The figure shows three views and two pictorial views of one solid part (mm, origin at its lowest corner). Answer the questions. A direction names the side the tool comes from. Round coordinates to 2 decimals unless told otherwise and drop trailing zeros. Write each loop counter-clockwise with the first axis right and the second up, starting at its lowest first coordinate (ties: lowest second). Pieces come first, ordered by that corner, then holes. Notation, with made-up numbers: M 83.25,33 L 134.25,33 A25 cw 134.25,46 Z; hole C 49,58 d7. An arc over 180 degrees is marked long. Answer in a Markdown table with one row per item.
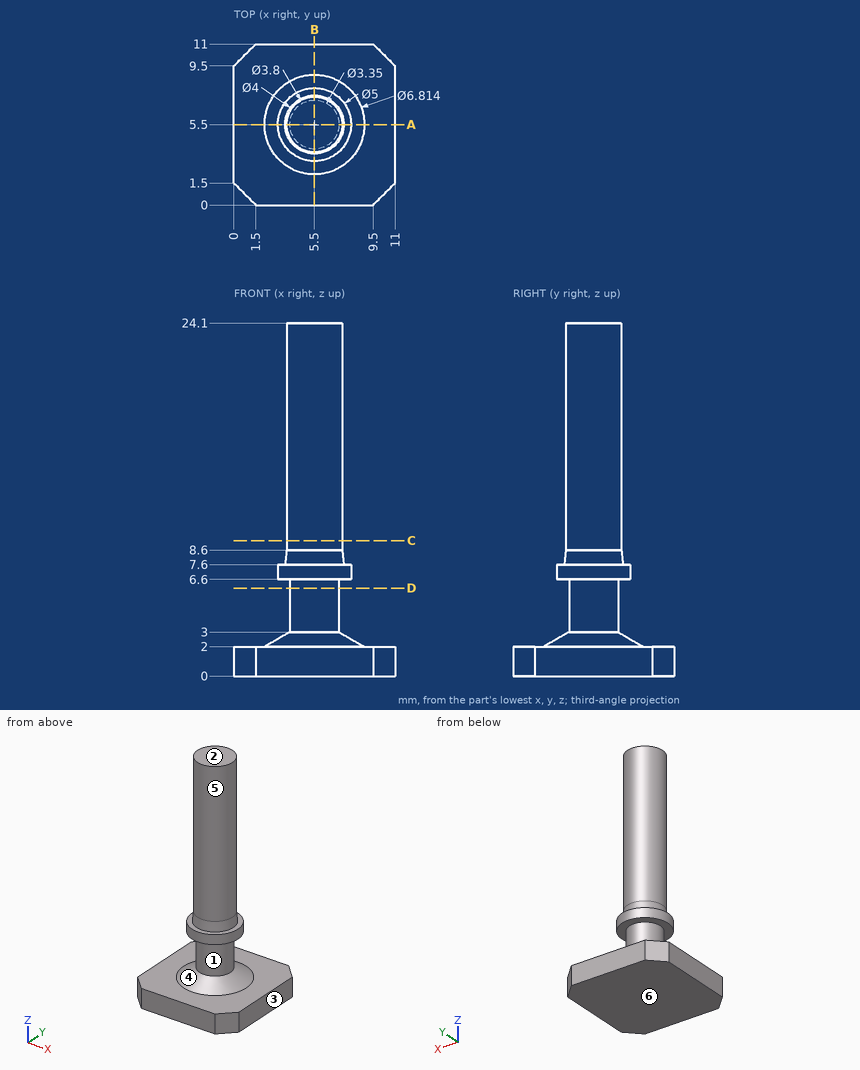
1. A tool of negligible diameter and unlimited length cuts with its end or side. For the marked faces 4, 5 and 6, from which of +Z, -Z, +X, -X, +Y, -Y can it reach the whole face along a straight path? Write none if from no direction.
Calculated:
| item | result |
|---|---|
| face 4 | none |
| face 5 | +Z |
| face 6 | -Z, +X, -X, +Y, -Y |
2. Determine the mould class of the marked faces 1, 2 and 3 for opening direction Z: released by +Z, released by -Z, zero draft, split by the parting line, or undercut.
Calculated:
| item | result |
|---|---|
| face 1 | undercut |
| face 2 | released by +Z |
| face 3 | zero draft |
3. Given pin 1 (1.5 mm diameter, centred on x = 3, y = 8.5, fed in from +Z); pin 2 (5 mm diameter, centred on x = 9.5, z = 14.5, fed in from -Y); pin 3 (5 mm diameter, centred on x = 8, z = 19, fed in from +Y), each flat-ended and moving along its own axis, determine where each tip first touches the part or whether it passes through.
Calculated:
| item | result |
|---|---|
| pin 1 | stops at z = 2.15 |
| pin 2 | stops at y = 4.33 |
| pin 3 | stops at y = 7.4 |
4. The part is cut by section A-A (y = 5.5). Determine the outline of the cut face in (x, z) (3 decimals).
Calculated:
| item | result |
|---|---|
| outline | M 0,0 L 11,0 L 11,2 L 8.907,2 L 7.175,3 L 7.175,6.6 L 8,6.6 L 8,7.6 L 7.5,7.6 L 7.4,8.6 L 7.4,24.1 L 3.6,24.1 L 3.6,8.6 L 3.5,7.6 L 3,7.6 L 3,6.6 L 3.825,6.6 L 3.825,3 L 2.093,2 L 0,2 Z |
5. The part is cut by section D-D (z = 6). Determine the outline of the cut face in (x, y) (3 decimals).
Calculated:
| item | result |
|---|---|
| outline | C 5.5,5.5 d3.35 |
6. The part is cut by section C-C (z = 9.25). Determine the outline of the cut face in (x, y).
Calculated:
| item | result |
|---|---|
| outline | C 5.5,5.5 d3.8 |
7. Consider line 1 along Z through (x, y) = (1.25, 9.25); line 2 along Z through (x, y) = (3, 7.25) (1 decimal); line 3 along Y through (x, z) = (6.5, 17.25). Determine where each line is inside the solid, lowest interval first. Write a range as from..to.
Calculated:
| item | result |
|---|---|
| line 1 | z = 0..2 |
| line 2 | z = 0..2.2 |
| line 3 | y = 3.88..7.12 |
